Autodesk Inventor part; units mm, degrees
ref_plane "to_block1_XY" through (0, -3.25, 0) normal (0, 0, 1) x (1, 0, 0)
ref_plane "to_block1_YZ" through (0, -3.25, 0) normal (1, 0, 0) x (0, 1, 0)
ref_plane "to_block1_ZX" through (0, -3.25, 0) normal (0, 1, 0) x (0, 0, 1)
sketch "_____1" plane through (0, 0, 0) normal (0, 0, 1) x (1, 0, 0)
  line L0 (-4.5, 2.95) -> (-4.5, 2.1665)
  arc A0 (-3.9835, 1.65) -> (-4.5, 2.1665) centre (-4.9, 1.25) ccw
  line L1 (-3.9835, 1.65) -> (-3.6, 1.65)
  arc A1 (-3.6, 0.85) -> (-3.6, 1.65) centre (-3.6, 1.25) ccw
  line L2 (-3.6, 0.85) -> (-3.9835, 0.85)
  arc A2 (-4.5, 0.3335) -> (-3.9835, 0.85) centre (-4.9, 1.25) ccw
  line L3 (-4.5, 0.3335) -> (-4.5, -2.95)
  line L4 (-4.5, -2.95) -> (-4.2, -3.25)
  line L5 (-4.2, -3.25) -> (4.2, -3.25)
  line L6 (4.2, -3.25) -> (4.5, -2.95)
  line L7 (4.5, -2.95) -> (4.5, 0.3335)
  arc A3 (3.9835, 0.85) -> (4.5, 0.3335) centre (4.9, 1.25) ccw
  line L8 (3.9835, 0.85) -> (3.6, 0.85)
  arc A4 (3.6, 1.65) -> (3.6, 0.85) centre (3.6, 1.25) ccw
  line L9 (3.6, 1.65) -> (3.9835, 1.65)
  arc A5 (4.5, 2.1665) -> (3.9835, 1.65) centre (4.9, 1.25) ccw
  line L10 (4.5, 2.1665) -> (4.5, 2.95)
  line L11 (4.5, 2.95) -> (4.2, 3.25)
  line L12 (4.2, 3.25) -> (-4.2, 3.25)
  line L13 (-4.2, 3.25) -> (-4.5, 2.95)
extrude "Extrusion1" add sketch "_____1" along normal mid plane 115
sketch "_____5" plane through (0, 0, 50) normal (0, 0, 1) x (1, 0, 0)
  line L0 (0, 3.25) -> (0, -3.25)
  line L1 (0, -3.25) -> (-2.1, -3.25)
  line L2 (-2.1, -3.25) -> (-1.8, -2.95)
  line L3 (-1.8, -2.95) -> (-1.8, -0.25)
  line L4 (-1.8, -0.25) -> (-3, -0.25)
  line L5 (-3, -0.25) -> (-3, 2.95)
  line L6 (-3, 2.95) -> (-3.3, 3.25)
  line L7 (-3.3, 3.25) -> (0, 3.25)
  line L8 (0, 3.25) -> (0, -3.25)
revolve "Revolution1" cut sketch "_____5" angle 360 about axis through (0, 3.25, 50) along (0, 1, 0)
pattern_linear "Rectangular Pattern1" count 6 spacing 20 along (0, 0, -1) of "Revolution1"
ref_plane "to_block1_XY" through (0, -3.25, 0) normal (0, 0, 1) x (1, 0, 0)
ref_plane "to_block1_YZ" through (0, -3.25, 0) normal (1, 0, 0) x (0, 1, 0)
ref_plane "to_block1_ZX" through (0, -3.25, 0) normal (0, 1, 0) x (0, 0, 1)
properties part number "C-MLG9-115_r"
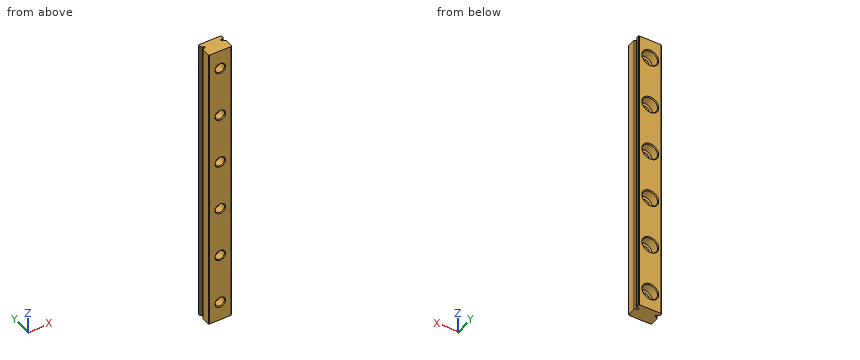
Source: CAD feature listing. Evaluate the final solid. Frame: model axes, mm. Give positions to 0.01 mm unless a question says otherwise; leave off trailing zeros. Loops run counter-clockwise (first coordinate to the right, second up) from the corner with the lowest first, then second, coordinate; pieces in that order, holes last. Notation, with made-up numbers: (40.25, 51.25) - (60.25, 51.25) arc R5 ccw to (60.25, 55.25) - close; hole circle Ø1 at (0, -2.75). An arc over 180 degrees is marked (long way). Use CSV: the item, a comma, the result in double quotes.
1) Pin query (flat end, axial travel): P1, Ø2, axis at x = 0, z = 50, coming from the -Y side; P2, Ø3, axis at x = 0.5, z = 31, coming from the +Y side. Return the tip coordinate at first contact, or that it passes through.
Worked out:
P1,"passes through"
P2,"stops at y = -0.25"
2) Cut plane C-C (z = -24). Output: boundary loops of the cut face in (x, y).
Worked out:
outline,"(-4.5, -2.95) - (-4.2, -3.25) - (4.2, -3.25) - (4.5, -2.95) - (4.5, 0.33) arc R1 cw to (3.98, 0.85) - (3.6, 0.85) arc R0.4 cw to (3.6, 1.65) - (3.98, 1.65) arc R1 cw to (4.5, 2.17) - (4.5, 2.95) - (4.2, 3.25) - (-4.2, 3.25) - (-4.5, 2.95) - (-4.5, 2.17) arc R1 cw to (-3.98, 1.65) - (-3.6, 1.65) arc R0.4 cw to (-3.6, 0.85) - (-3.98, 0.85) arc R1 cw to (-4.5, 0.33) - close"
3) Line query: line 1 (Y direction, x = 2.25, z = 31.5); line 2 (X direction, y = 1.5, z = -30.5); line 3 (X direction, y = 0.25, z = -9.5). Output: solid intervals per line, ascending.
Worked out:
line 1,"y = -3.25 to -0.25"
line 2,"x = -3.29 to -2.96, 2.96 to 3.29"
line 3,"x = -4.5 to -2.96, 2.96 to 4.5"
4) Cut plane B-B (x = 0). Count the separate pieces of the cut face and the enclosed holes in it, and give its area (3 significant figures).
Worked out:
separate pieces,"7"
enclosed holes,"0"
area,"556 mm^2"
